CAD build for the part. Positions are in the model's coordinates, mm. A direction names the side the tool comes from. Give positions to 0.01 mm unless a question says otherwise; leave off trailing zeros. Write each loop counter-clockwise with the first axis right and the second up, starting at its lowest first coordinate (ties: lowest second). Pieces come first, ordered by that corner, then holes. Notation, with made-up numbers: (14, 56) -> (71, 56) arc R33 cw to (71, 89) -> close; hole circle Ø7 at (40, 57.25). An arc over 180 degrees is marked (long way). Use one line per item in the form item = value. Start each with the question number.
from build123d import *

# Parameters (mm, degrees)
SKETCH2_W          = 4
SKETCH2_H          = 7
CUT_EXTRUDE1_DEPTH = 40


with BuildPart() as part:
    # Sketch1 → Revolve1 (revolve)
    with BuildSketch(Plane.XY):
        with BuildLine():
            Line((16, 30), (17, 30))
            ThreePointArc((17, 30), (18.414213562, 29.414213562), (19, 28))
            Line((19, 28), (19, 12))
            ThreePointArc((19, 12), (19.585786438, 10.585786438), (21, 10))
            Line((21, 10), (25, 10))
            Line((25, 10), (25, 5))
            Line((25, 5), (0, 5))
            Line((0, 5), (0, 28))
            ThreePointArc((0, 28), (0.585786438, 29.414213562), (2, 30))
            Line((2, 30), (3, 30))
            Line((3, 30), (5.911761874, 22))
            Line((5.911761874, 22), (13.088238126, 22))
            Line((13.088238126, 22), (16, 30))
        make_face()
    revolve(axis=Axis((-3.782421274, 0, 0), (1, 0, 0)))

    # Sketch2 → Cut-Extrude1 (cut)
    with BuildSketch(Plane(origin=(25, 0, 0), x_dir=(0, 0, -1), z_dir=(1, 0, 0))):
        with Locations((0, 3.5)):
            Rectangle(SKETCH2_W, SKETCH2_H)
    extrude(amount=-CUT_EXTRUDE1_DEPTH, mode=Mode.SUBTRACT)


solid = part.part
1) 3-axis set-ups, long thin cutter, end or side, ignore diameter. For faces 4 (the face through (23.03, -2.17, -9.76)), 5 (the face through (25, -5, -2)), 6 (the face through (13.27, -4.878, -21.965)), 7 (the face through (13, 6, 2)): which of +Z, -Z, +X, -X, +Y, -Y reach the whole face in a straight line?
2) Wall check: line 1 along Z through (x, y) = (8, 0); line 2 along Y through (x, z) = (21.5, 3); line 3 along X through (y, z) = (-23, -9.5). Give the ranges that are in metal, low to high. Write a range as from..to.
3) Pin check, flat tips, straight feed: pin 1 (2.5 mm diameter, centred on x = 16, y = 6, fed in from -Z); pin 2 (2 mm diameter, centred on x = 2.5, z = -14.5, fed in from +Y); pin 3 (2 mm diameter, centred on x = 7, z = 0, fed in from -Y). Stop position of each tip, or through.
4) Cut at B-B (x = 22.25). Give the cut face in (y, z), and give its area (3 significant figures).
5) Two-plate mould, pull along X, no slides. Class faces 1 (the face through (12, -5, 0)), 2 (the face through (9.55, -4.769, -21.477)), 3 (the face through (0, -6, 0)): released by +X, released by -X, zero draft, split by the parting line, or undercut.
6) Cut at A-A (y = 0). Give the cut face in (x, z), and give its area (3 significant figures).
7) Cut at C-C (z = 0). Give the cut face in (x, y), and give its area (3 significant figures).
Final values:
q1.face_4 = +X
q1.face_5 = +Z, -Z, +X, +Y, -Y
q1.face_6 = none
q1.face_7 = +X, -X
q2.line_1 = -22..-5, 5..22
q2.line_2 = -9.54..-4, 4..9.54
q2.line_3 = 0..4.86, 14.14..19
q3.pin_1 = -29.62
q3.pin_2 = 26.79
q3.pin_3 = -22
q4.outline = circle Ø20 at (0, 0); hole (4.58, -2) -> (7, -2) -> (7, 2) -> (4.58, 2) arc R5 ccw (long way) to start
q4.area = 227 mm^2
q5.face_1 = zero draft
q5.face_2 = undercut
q5.face_3 = released by -X
q6.outline = (0, -28) arc R2 ccw to (2, -30) -> (3, -30) -> (5.91, -22) -> (13.09, -22) -> (16, -30) -> (17, -30) arc R2 ccw to (19, -28) -> (19, -12) arc R2 cw to (21, -10) -> (25, -10) -> (25, -5) -> (0, -5) -> close; (0, 5) -> (25, 5) -> (25, 10) -> (21, 10) arc R2 cw to (19, 12) -> (19, 28) arc R2 ccw to (17, 30) -> (16, 30) -> (13.09, 22) -> (5.91, 22) -> (3, 30) -> (2, 30) arc R2 ccw to (0, 28) -> close
q6.area = 847 mm^2
q7.outline = (0, -28) arc R2 ccw to (2, -30) -> (3, -30) -> (5.91, -22) -> (13.09, -22) -> (16, -30) -> (17, -30) arc R2 ccw to (19, -28) -> (19, -12) arc R2 cw to (21, -10) -> (25, -10) -> (25, -5) -> (0, -5) -> close; (0, 7) -> (25, 7) -> (25, 10) -> (21, 10) arc R2 cw to (19, 12) -> (19, 28) arc R2 ccw to (17, 30) -> (16, 30) -> (13.09, 22) -> (5.91, 22) -> (3, 30) -> (2, 30) arc R2 ccw to (0, 28) -> close
q7.area = 797 mm^2
